Read the model definition and answer for the solid it produces. Units are mm, in the model's axes. Coordinates: 2 decimals unless noted, no trailing zeros. Loops run counter-clockwise (first coordinate to the right, second up) from the corner with the lowest first, then second, coordinate; pieces in that order, holes last.
Autodesk Fusion 360 part; units mm, degrees
sketch "Sketch2" plane through (0, 0, 0) normal (0, 0, 1) x (1, 0, 0)
sketch "Sketch3" plane through (0, 0, 0) normal (0, 1, 0) x (1, 0, 0)
  line L0 (85.725, 0) -> (101.6, 0)
  line L1 (88.9, -50.8) -> (85.725, -50.8)
  line L2 (187.325, -12.7) -> (184.15, -12.7)
  line L3 (104.4448, -12.7) -> (104.4448, -9.525)
  line L4 (88.9, -12.7) -> (85.725, -12.7)
  line L5 (85.725, -25.4) -> (85.725, -12.7)
  line L6 (91.7448, -12.7) -> (104.4448, -12.7)
  line L7 (88.9, -63.5) -> (88.9, -50.8)
  line L8 (181.3052, -12.7) -> (168.6052, -12.7)
  line L9 (88.9, -76.2) -> (88.9, -63.5)
  line L10 (181.3052, -53.975) -> (91.7448, -53.975)
  line L11 (85.725, 0) -> (87.3125, 0)
  line L12 (91.7448, 0) -> (91.7448, -12.7)
  line L13 (88.9, -50.8) -> (88.9, -38.1)
  line L14 (88.9, -25.4) -> (88.9, -12.7)
  line L15 (176.2252, 0) -> (181.3052, 0)
  line L16 (187.325, -38.1) -> (184.15, -38.1)
  line L17 (158.4452, -12.7) -> (156.5402, -12.7)
  line L18 (96.8248, -12.7) -> (104.4448, -12.7)
  line L19 (168.6052, -12.7) -> (176.2252, -12.7)
  line L20 (91.7448, -12.7) -> (96.8248, -12.7)
  line L21 (88.9, -38.1) -> (88.9, -25.4)
  line L22 (168.6052, -12.7) -> (168.6052, -9.525)
  line L23 (96.8248, 0) -> (91.7448, 0)
  line L24 (187.325, -25.4) -> (184.15, -25.4)
  line L25 (88.9, -25.4) -> (85.725, -25.4)
  line L26 (114.6048, -12.7) -> (156.5402, -12.7)
  line L27 (158.4452, -9.525) -> (158.4452, -12.7)
  line L28 (114.6048, -9.525) -> (114.6048, -12.7)
  line L29 (187.325, 0) -> (187.325, -12.7)
  line L30 (181.3052, -12.7) -> (176.2252, -12.7)
  line L31 (187.325, 0) -> (184.15, 0)
  line L32 (85.725, 0) -> (96.8248, 0)
  line L33 (187.325, 0) -> (176.2252, 0)
  line L34 (184.15, -12.7) -> (184.15, 0)
  line L35 (184.15, -25.4) -> (184.15, -12.7)
  line L36 (88.9, -139.7) -> (85.725, -139.7)
  line L37 (88.9, -101.6) -> (88.9, -95.25)
  line L38 (88.9, -127) -> (85.725, -127)
  line L39 (88.9, -95.25) -> (88.9, -88.9)
  line L40 (184.15, -101.6) -> (184.15, -88.9)
  line L41 (88.9, -114.3) -> (88.9, -101.6)
  line L42 (187.325, -101.6) -> (187.325, -114.3)
  line L43 (184.15, -127) -> (184.15, -114.3)
  line L44 (88.9, -127) -> (88.9, -114.3)
  line L45 (187.325, -101.6) -> (184.15, -101.6)
  line L46 (187.325, -139.7) -> (187.325, -127)
  line L47 (184.15, -139.7) -> (187.325, -139.7)
  line L48 (88.9, -114.3) -> (85.725, -114.3)
  line L49 (88.9, -139.7) -> (88.9, -127)
  line L50 (187.325, -114.3) -> (187.325, -101.6)
  line L51 (187.325, -127) -> (184.15, -127)
  line L52 (88.9, -88.9) -> (85.725, -88.9)
  line L53 (91.7448, -97.155) -> (181.3052, -97.155)
  line L54 (85.725, -101.6) -> (85.725, -88.9)
  line L55 (88.9, -101.6) -> (85.725, -101.6)
  line L56 (187.325, -127) -> (187.325, -139.7)
  line L57 (184.15, -88.9) -> (187.325, -88.9)
  line L58 (184.15, -114.3) -> (187.325, -114.3)
  line L59 (85.725, -127) -> (85.725, -114.3)
  line L60 (184.15, 0) -> (184.15, -203.2)
  line L61 (85.725, -203.2) -> (88.9, -203.2)
  line L62 (88.9, 0) -> (88.9, -203.2)
  line L63 (88.9, -165.1) -> (88.9, -152.4)
  line L64 (187.325, -152.4) -> (187.325, -165.1)
  line L65 (184.15, -203.2) -> (184.15, -190.5)
  line L66 (184.15, -152.4) -> (184.15, -139.7)
  line L67 (88.9, -203.2) -> (88.9, -190.5)
  line L68 (85.725, -152.4) -> (85.725, -139.7)
  line L69 (88.9, -165.1) -> (85.725, -165.1)
  line L70 (88.9, -190.5) -> (85.725, -190.5)
  line L71 (88.9, -177.8) -> (85.725, -177.8)
  line L72 (184.15, -177.8) -> (187.325, -177.8)
  line L73 (184.15, -190.5) -> (184.15, -177.8)
  line L74 (88.9, -152.4) -> (88.9, -139.7)
  line L75 (184.15, -165.1) -> (187.325, -165.1)
  line L76 (187.325, -177.8) -> (187.325, -190.5)
  line L77 (88.9, -152.4) -> (85.725, -152.4)
  line L78 (187.325, -152.4) -> (184.15, -152.4)
  line L79 (184.15, -190.5) -> (187.325, -190.5)
  line L80 (184.15, -76.2) -> (187.325, -76.2)
  line L81 (181.3052, 0) -> (181.3052, -12.7)
  line L82 (91.7448, -59.055) -> (181.3052, -59.055)
  line L83 (187.325, -165.1) -> (187.325, -152.4)
  line L84 (91.7448, -59.055) -> (91.7448, -97.155)
  line L85 (88.9, -63.5) -> (85.725, -63.5)
  line L86 (184.15, -177.8) -> (184.15, -165.1)
  line L87 (184.15, -50.8) -> (184.15, -38.1)
  line L88 (85.725, 0) -> (187.325, 0)
  line L89 (184.15, -63.5) -> (187.325, -63.5)
  line L90 (187.325, -25.4) -> (187.325, -38.1)
  line L91 (187.325, 0) -> (175.26, 0)
  line L92 (184.15, -76.2) -> (184.15, -63.5)
  line L93 (181.3052, -59.055) -> (181.3052, -97.155)
  line L94 (187.325, -50.8) -> (187.325, -63.5)
  line L95 (168.6052, -9.525) -> (158.4452, -9.525)
  line L96 (184.15, -38.1) -> (184.15, -25.4)
  line L97 (85.725, -76.2) -> (85.725, -63.5)
  line L98 (85.725, -177.8) -> (85.725, -165.1)
  line L99 (91.7448, -12.7) -> (91.7448, -53.975)
  line L100 (85.725, -50.8) -> (85.725, -38.1)
  line L101 (104.4448, -9.525) -> (114.6048, -9.525)
  line L102 (184.15, -50.8) -> (187.325, -50.8)
  line L103 (88.9, -177.8) -> (88.9, -165.1)
  line L104 (181.3052, -12.7) -> (181.3052, -53.975)
  line L105 (187.325, -76.2) -> (187.325, -88.9)
  line L106 (88.9, -190.5) -> (88.9, -177.8)
  line L107 (184.15, -88.9) -> (184.15, -76.2)
  line L108 (184.15, -203.2) -> (85.725, -203.2)
  line L109 (88.9, -76.2) -> (85.725, -76.2)
  line L110 (88.9, -88.9) -> (88.9, -76.2)
  line L111 (88.9, -38.1) -> (85.725, -38.1)
  line L112 (85.725, 0) -> (88.9, 0)
  line L113 (91.7448, -53.975) -> (91.7448, -59.055)
  line L114 (85.725, -203.2) -> (85.725, -190.5)
  line L115 (184.15, -63.5) -> (184.15, -50.8)
  point P0 (187.325, 0)
  dimension "d68" = 11.0998
  dimension "d69" = 11.0998
  dimension "d70" = 12.7
  dimension "d71" = 12.7
  dimension "d72" = 5.08
  dimension "d73" = 5.08
  dimension "d74" = 41.275
  dimension "d75" = 5.08
  dimension "d76" = 5.08
  dimension "d77" = 38.1
  dimension "d78" = 3.175
  dimension "d79" = 3.175
  dimension "d80" = 3.175
  dimension "d81" = 3.175
  dimension "d82" = 12.7
  dimension "d83" = 12.7
  dimension "d84" = 12.7
  dimension "d85" = 12.7
  dimension "d86" = 12.7
  dimension "d87" = 12.7
  dimension "d88" = 12.7
  dimension "d89" = 12.7
  dimension "d90" = 6.35
  dimension "d91" = 6.35
  dimension "d92" = 12.7
  dimension "d93" = 12.7
  dimension "d94" = 12.7
  dimension "d95" = 12.7
  dimension "d96" = 12.7
  dimension "d97" = 12.7
  dimension "d98" = 12.7
  dimension "d99" = 12.7
  dimension "d100" = 3.175
  dimension "d101" = 10.16
  dimension "d102" = 3.175
  dimension "d103" = 10.16
extrude "Extrude1" add sketch "Sketch3" along normal blind 3.175 contours L0 L7 L9 L10 L12 L13 L14 L21 L32 L33 L34 L35 L37 L39 L40 L41 L43 L44 L49 L60 L62 L63 L65 L66 L67 L73 L74 L81 L86 L87 L88 L91 L92 L96 L99 L103 L104 L106 L107 L108 L110 L115 | L0 L3 L6 L8 L12 L15 L17 L18 L19 L20 L22 L23 L26 L27 L28 L30 L32 L33 L81 L88 L91 L95 L101 | L4 L5 L14 L25 L62 | L1 L13 L62 L100 L111 | L9 L62 L85 L97 L109 | L2 L29 L31 L33 L34 L60 L88 L91 | L37 L39 L52 L54 L55 L62 | L16 L24 L60 L90 L96 | L38 L44 L48 L59 L62 | L60 L89 L94 L102 L115 | L36 L62 L68 L74 L77 | L57 L60 L80 L105 L107 | L62 L69 L71 L98 L103 | L42 L45 L50 L58 L60 | L61 L62 L67 L70 L108 L114 | L46 L47 L51 L56 L60 | L60 L64 L75 L78 L83 | L60 L72 L73 L76 L79
sketch "Sketch4" plane through (0, 0, 0) normal (0, -1, 0) x (1, 0, 0)
  line L0 (168.6052, 12.7) -> (168.6052, 9.525)
  line L1 (168.6052, 9.525) -> (158.4452, 9.525)
  line L2 (158.4452, 9.525) -> (158.4452, 12.7)
  line L3 (158.4452, 12.7) -> (156.5402, 12.7)
  line L4 (156.5402, 12.7) -> (114.6048, 12.7)
  line L5 (114.6048, 12.7) -> (114.6048, 9.525)
  line L6 (114.6048, 9.525) -> (104.4448, 9.525)
  line L7 (104.4448, 9.525) -> (104.4448, 12.7)
  line L8 (104.4448, 12.7) -> (96.8248, 12.7)
  line L9 (96.8248, 12.7) -> (91.7448, 12.7)
  line L10 (91.7448, 12.7) -> (91.7448, 53.975)
  line L11 (91.7448, 53.975) -> (181.3052, 53.975)
  line L12 (181.3052, 53.975) -> (181.3052, 12.7)
  line L13 (181.3052, 12.7) -> (176.2252, 12.7)
  line L14 (176.2252, 12.7) -> (168.6052, 12.7)
  line L15 (91.7448, 59.055) -> (91.7448, 97.155)
  line L16 (91.7448, 97.155) -> (181.3052, 97.155)
  line L17 (181.3052, 97.155) -> (181.3052, 59.055)
  line L18 (181.3052, 59.055) -> (91.7448, 59.055)
  line L19 (184.15, 190.5) -> (184.15, 203.2)
  line L20 (184.15, 203.2) -> (85.725, 203.2)
  line L21 (85.725, 203.2) -> (85.725, 190.5)
  line L22 (85.725, 190.5) -> (88.9, 190.5)
  line L23 (88.9, 190.5) -> (88.9, 177.8)
  line L24 (88.9, 177.8) -> (85.725, 177.8)
  line L25 (85.725, 177.8) -> (85.725, 165.1)
  line L26 (85.725, 165.1) -> (88.9, 165.1)
  line L27 (88.9, 165.1) -> (88.9, 152.4)
  line L28 (88.9, 152.4) -> (85.725, 152.4)
  line L29 (85.725, 152.4) -> (85.725, 139.7)
  line L30 (85.725, 139.7) -> (88.9, 139.7)
  line L31 (88.9, 139.7) -> (88.9, 127)
  line L32 (88.9, 127) -> (85.725, 127)
  line L33 (85.725, 127) -> (85.725, 114.3)
  line L34 (85.725, 114.3) -> (88.9, 114.3)
  line L35 (88.9, 114.3) -> (88.9, 101.6)
  line L36 (88.9, 101.6) -> (85.725, 101.6)
  line L37 (85.725, 101.6) -> (85.725, 88.9)
  line L38 (85.725, 88.9) -> (88.9, 88.9)
  line L39 (88.9, 88.9) -> (88.9, 76.2)
  line L40 (88.9, 76.2) -> (85.725, 76.2)
  line L41 (85.725, 76.2) -> (85.725, 63.5)
  line L42 (85.725, 63.5) -> (88.9, 63.5)
  line L43 (88.9, 63.5) -> (88.9, 50.8)
  line L44 (88.9, 50.8) -> (85.725, 50.8)
  line L45 (85.725, 50.8) -> (85.725, 38.1)
  line L46 (85.725, 38.1) -> (88.9, 38.1)
  line L47 (88.9, 38.1) -> (88.9, 25.4)
  line L48 (88.9, 25.4) -> (85.725, 25.4)
  line L49 (85.725, 25.4) -> (85.725, 12.7)
  line L50 (85.725, 12.7) -> (88.9, 12.7)
  line L51 (88.9, 12.7) -> (88.9, 0)
  line L52 (88.9, 0) -> (187.325, 0)
  line L53 (187.325, 0) -> (187.325, 12.7)
  line L54 (187.325, 12.7) -> (184.15, 12.7)
  line L55 (184.15, 12.7) -> (184.15, 25.4)
  line L56 (184.15, 25.4) -> (187.325, 25.4)
  line L57 (187.325, 25.4) -> (187.325, 38.1)
  line L58 (187.325, 38.1) -> (184.15, 38.1)
  line L59 (184.15, 38.1) -> (184.15, 50.8)
  line L60 (184.15, 50.8) -> (187.325, 50.8)
  line L61 (187.325, 50.8) -> (187.325, 63.5)
  line L62 (187.325, 63.5) -> (184.15, 63.5)
  line L63 (184.15, 63.5) -> (184.15, 76.2)
  line L64 (184.15, 76.2) -> (187.325, 76.2)
  line L65 (187.325, 76.2) -> (187.325, 88.9)
  line L66 (187.325, 88.9) -> (184.15, 88.9)
  line L67 (184.15, 88.9) -> (184.15, 101.6)
  line L68 (184.15, 101.6) -> (187.325, 101.6)
  line L69 (187.325, 101.6) -> (187.325, 114.3)
  line L70 (187.325, 114.3) -> (184.15, 114.3)
  line L71 (184.15, 114.3) -> (184.15, 127)
  line L72 (184.15, 127) -> (187.325, 127)
  line L73 (187.325, 127) -> (187.325, 139.7)
  line L74 (187.325, 139.7) -> (184.15, 139.7)
  line L75 (184.15, 139.7) -> (184.15, 152.4)
  line L76 (184.15, 152.4) -> (187.325, 152.4)
  line L77 (187.325, 152.4) -> (187.325, 165.1)
  line L78 (187.325, 165.1) -> (184.15, 165.1)
  line L79 (184.15, 165.1) -> (184.15, 177.8)
  line L80 (184.15, 177.8) -> (187.325, 177.8)
  line L81 (187.325, 177.8) -> (187.325, 190.5)
  line L82 (187.325, 190.5) -> (184.15, 190.5)
  line L83 (88.9, 0) -> (104.14, 0)
  line L84 (168.6052, 9.525) -> (168.6052, 0)
  line L85 (168.6052, 0) -> (187.325, 0)
  line L86 (104.4448, 9.525) -> (104.4448, 0)
equation "d68 = 0.5 in - 0.063 in"
equation "d74 = 1.5 in + 0.125 in"
Q1. Flat-ended cylindrical pins translate along their axes: pin 1 Ø1.5 at (y, z) = (2.5, 56.5) entering from -X; pin 2 Ø1 at (y, z) = (2, 145.5) entering from +X. Find the tip coordinate at first contact, or state that the pin passes through.
Findings below:
pin 1: stops at x = 88.9
pin 2: stops at x = 184.15
Q2. Straight lines are drawn through the part: probe 1 along Z at (x, y) = (119, 1.7) (3 decimals); probe 2 along Z at (x, y) = (159, 2.95) (3 decimals); probe 3 along X at (y, z) = (2.15, 66) (3 decimals). For each, find the intervals that lie inside material, in ascending order.
Findings below:
probe 1: z = 0 to 12.7, 53.975 to 59.055, 97.155 to 203.2
probe 2: z = 0 to 9.525, 53.975 to 59.055, 97.155 to 203.2
probe 3: x = 85.725 to 91.745, 181.305 to 184.15
Q3. A cutting plane is placed at C-C (y = 1.6). Count the separate pieces of the cut face and the enclosed holes in it, then the cut area to 3 significant figures.
Findings below:
separate pieces: 1
enclosed holes: 2
area: 12,800 mm2
Q4. A cutting plane is placed at A-A (x = 166). Give the vertices of the cut face in (y, z) (3 decimals), then the cut area to 3 significant figures.
Findings below:
outline: (0, 0) - (3.175, 0) - (3.175, 9.525) - (0, 9.525) - close; (0, 53.975) - (3.175, 53.975) - (3.175, 59.055) - (0, 59.055) - close; (0, 97.155) - (3.175, 97.155) - (3.175, 203.2) - (0, 203.2) - close
area: 383 mm2
Q5. A cutting plane is placed at B-B (z = 91.5). Give the vertices of the cut face in (x, y) (3 decimals), then the cut area to 3 significant figures.
Findings below:
outline: (85.725, 0) - (91.745, 0) - (91.745, 3.175) - (85.725, 3.175) - close; (181.305, 0) - (184.15, 0) - (184.15, 3.175) - (181.305, 3.175) - close
area: 28.1 mm2
Q6. A cutting plane is placed at D-D (z = 131.5). Give the vertices of the cut face in (x, y) (3 decimals).
Findings below:
outline: (88.9, 0) - (187.325, 0) - (187.325, 3.175) - (88.9, 3.175) - close
